```python
from build123d import *

# Parameters (mm, degrees)
F0_R     = 11
F1_DEPTH = 20
F2_R     = 10
F3_DEPTH = 14
F5_DEPTH = 75
F6_R     = 3.2
F6_R_2   = 3.25
F7_DEPTH = 12.5


with BuildPart() as f1:
    # F0 (on Right) → F1 (new body)
    with BuildSketch(Plane.YZ):
        Circle(F0_R)
    extrude(amount=F1_DEPTH)

    # F2 (on face) → F3 (cut)
    with BuildSketch(Plane(origin=(0, 0, 0), x_dir=(0, -1, 0), z_dir=(-1, 0, 0))):
        Circle(F2_R)
    extrude(amount=-F3_DEPTH, mode=Mode.SUBTRACT)

    # F4 (on face) → F5 (join)
    with BuildSketch(Plane.YZ.offset(20)):
        with BuildLine():
            Line((0, -11), (0, 11))
            ThreePointArc((0, 11), (-11, 0), (0, -11))
        make_face()
    extrude(amount=F5_DEPTH)

    # F6 (on Front) → F7 (cut, symmetric)
    with BuildSketch(Plane.XZ):
        with Locations((9, 0)):
            Circle(F6_R)
        with Locations((90, 0)):
            Circle(F6_R_2)
    extrude(amount=F7_DEPTH, both=True, mode=Mode.SUBTRACT)


solid = f1.part
```
Design review of the part built by this model. Coordinates are the model's own, in mm. A direction names the side the tool comes from. Round coordinates to 2 decimals unless told otherwise and drop trailing zeros. Order: outer loops, then holes, each group sorted by start corner. A loop starts at its lowest first (then second) coordinate and runs counter-clockwise, first axis right, second up. Notation, with made-up numbers: M 27.5,-31.75 L 39.5,-31.75 A20 cw 39.5,-23.75 Z; hole C 29,49.5 d9. An arc over 180 degrees is marked long. Put each result on its own line as item: value.
Q1. Machinability: for faces 1 (the face through (5.8, 10.2, 0.1)), 2 (the face through (20, 4, 0)), 3 (the face through (6.902, -9.237, -3.83)), which of the approach directions +Z, -Z, +X, -X, +Y, -Y give a long, thin tool a straight path to every point of the face, cutting with its end or side? Answer none if there is none.
Reported:
face 1: +Y, -Y
face 2: +Z, -Z, +X, +Y
face 3: -X
Q2. To check wall thickness, follow line 1 (X direction, y = -6, z = 0); line 2 (X direction, y = 10.3, z = 0); line 3 (X direction, y = 2.75, z = 5.5). State the ranges of each line that lie inside material, in increasing order.
Reported:
line 1: 14 to 86.75, 93.25 to 95
line 2: 0 to 5.8, 12.2 to 20
line 3: 14 to 20
Q3. Draft analysis for pull direction X (two halves, no side actions). For faces 4 (the face through (14, 0, 0)), 5 (the face through (95, -4, 0)), 6 (the face through (86.753, -5.58, 0.143)), state which applies: released by +X, released by -X, zero draft, split by the parting line, or undercut.
Reported:
face 4: released by -X
face 5: released by +X
face 6: undercut
Q4. Consider section C-C (y = -2.5). State the section outline as (x, z) points.
Reported:
outline: M 0,-10.71 L 95,-10.71 L 95,10.71 L 0,10.71 L 0,9.68 L 14,9.68 L 14,-9.68 L 0,-9.68 Z; hole C 90,0 d6.5
Q5. Consider section D-D (z = 6.5). State the section outline as (x, y) points.
Reported:
outline: M 0,-8.87 L 95,-8.87 L 95,0 L 20,0 L 20,8.87 L 0,8.87 L 0,7.6 L 14,7.6 L 14,-7.6 L 0,-7.6 Z
Q6. Consider section A-A (z = 0). State the section outline as (x, y) points.
Reported:
outline: M 0,-11 L 5.8,-11 L 5.8,-10 L 0,-10 Z; M 0,10 L 5.8,10 L 5.8,11 L 0,11 Z; M 12.2,-11 L 86.75,-11 L 86.75,0 L 20,0 L 20,11 L 12.2,11 L 12.2,10 L 14,10 L 14,-10 L 12.2,-10 Z; M 93.25,-11 L 95,-11 L 95,0 L 93.25,0 Z
Q7. Consider section B-B (x = 88.5). State the section outline as (y, z) points, and give its area (3 significant figures).
Reported:
outline: M -10.62,-2.88 A11 ccw 0,-11 L 0,-2.88 Z; M -10.62,2.88 L 0,2.88 L 0,11 A11 ccw Z
area: 127 mm²
Q8. Insertion check: pin 1 Ø1 at (x, y) = (77, -3.5) entering from +Z; pin 2 Ø4 at (x, z) = (40, 6.5) entering from -Y; pin 3 Ø7.5 at (x, z) = (9, 0) entering from -Y; pin 4 Ø6 at (y, z) = (-3.5, -1) entering from -X. Each pin has a flat end and moves straight along its axis. Give the tip position at first contact, or say it passes through.
Reported:
pin 1: z = 10.58
pin 2: y = -10.04
pin 3: y = -11
pin 4: x = 14
